Geometry: final body of the model. Coordinates: model frame, mm. A direction names the side the tool comes from. Round coordinates to 2 decimals unless told otherwise and drop trailing zeros. Order: outer loops, then holes, each group sorted by start corner. A loop starts at its lowest first (then second) coordinate and runs counter-clockwise, first axis right, second up. Notation, with made-up numbers: (88, -5.5) - (103, -5.5) arc R13 cw to (103, 7.5) - close; hole circle Ø6 at (43, -9). An arc over 180 degrees is marked (long way). Put each result on its own line as item: value. Start each with the question number.
(1) Section D-D (x = -24.2). Output: boundary loops of the cut face in (y, z) (3 decimals).
(2) Pin query (flat end, axial travel): P1, Ø3, axis at x = 24.2, z = 19.7, coming from the -Y side. Return the tip coordinate at first contact, or that it passes through.
(3) Section A-A (x = -11.5). Output: boundary loops of the cut face in (y, z), and give its area (3 significant figures).
(4) Access query for faces 4 (the face through (-17.375, 1, 0)), 5 (the face through (0, 2, -19)). Directions: +Z, -Z, +X, -X, +Y, -Y. A direction counts if a zero-diameter tool reaches every point of the face in a straight line with its end or side. Return the directions, or none.
(5) Pull-direction query (Z, two-part tool) for faces 1 (the face through (22.59, 0.99, -20.93)), 2 (the face through (29.58, 0.99, 24.89)), 3 (the face through (-33, 1, 0)); classes: released by +Z, released by -Z, zero draft, split by the parting line, or undercut.
(6) Material intervals for L1, parallel to Z at x = 23, y = 1.5; L2, parallel to X at y = 1.2, z = -8.5 (3 decimals); L3, parallel to X at y = 0.6, z = 20, sorted ascending. Write a range as [from, to].
(7) Section B-B (y = 0.9). Output: boundary loops of the cut face in (x, z) (3 decimals), and give its area (3 significant figures).
(8) Section C-C (z = 12). Output: boundary loops of the cut face in (x, y) (3 decimals), and give its area (3 significant figures).
from build123d import *

# Parameters (mm, degrees)
F0_R     = 2.025
F0_W     = 34.75
F0_H     = 31.1
F1_DEPTH = 2


with BuildPart() as f1:
    # F0 (on Front) → F1 (new body)
    with BuildSketch(Plane.XZ):
        with BuildLine():
            Line((-21, -28.5), (21, -28.5))
            ThreePointArc((21, -28.5), (29.485281, -24.985281), (33, -16.5))
            Line((33, -16.5), (33, 16.5))
            ThreePointArc((33, 16.5), (29.485281, 24.985281), (21, 28.5))
            Line((21, 28.5), (-21, 28.5))
            ThreePointArc((-21, 28.5), (-29.485281, 24.985281), (-33, 16.5))
            Line((-33, 16.5), (-33, -16.5))
            ThreePointArc((-33, -16.5), (-29.485281, -24.985281), (-21, -28.5))
        make_face()
        with Locations((-24.2, -19.7)):
            Circle(F0_R, mode=Mode.SUBTRACT)
        with Locations((24.2, -19.7)):
            Circle(F0_R, mode=Mode.SUBTRACT)
        with Locations((-24.2, 19.7)):
            Circle(F0_R, mode=Mode.SUBTRACT)
        Rectangle(F0_W, F0_H, mode=Mode.SUBTRACT)
        with Locations((24.2, 19.7)):
            Circle(F0_R, mode=Mode.SUBTRACT)
    extrude(amount=-F1_DEPTH)


solid = f1.part
Checks:
1. outline: (0, -28.065) - (2, -28.065) - (2, -21.725) - (0, -21.725) - close; (0, -17.675) - (2, -17.675) - (2, 17.675) - (0, 17.675) - close; (0, 21.725) - (2, 21.725) - (2, 28.065) - (0, 28.065) - close
2. P1: passes through
3. outline: (0, -28.5) - (2, -28.5) - (2, -15.55) - (0, -15.55) - close; (0, 15.55) - (2, 15.55) - (2, 28.5) - (0, 28.5) - close
3. area: 51.8 mm²
4. face 4: +Y, -Y
4. face 5: +Z, -Z, +X, -X, +Y
5. face 1: undercut
5. face 2: released by +Z
5. face 3: zero draft
6. L1: z = [-28.33, -21.33], [-18.07, 18.07], [21.33, 28.33]
6. L2: x = [-33, -17.375], [17.375, 33]
6. L3: x = [-32.48, -26.2], [-22.2, 22.2], [26.2, 32.48]
7. outline: (-33, -16.5) arc R12 ccw to (-21, -28.5) - (21, -28.5) arc R12 ccw to (33, -16.5) - (33, 16.5) arc R12 ccw to (21, 28.5) - (-21, 28.5) arc R12 ccw to (-33, 16.5) - close; hole circle Ø4.05 at (-24.2, -19.7); hole circle Ø4.05 at (-24.2, 19.7); hole (-17.375, -15.55) - (17.375, -15.55) - (17.375, 15.55) - (-17.375, 15.55) - close; hole circle Ø4.05 at (24.2, -19.7); hole circle Ø4.05 at (24.2, 19.7)
7. area: 2,510 mm²
8. outline: (-33, 0) - (-17.375, 0) - (-17.375, 2) - (-33, 2) - close; (17.375, 0) - (33, 0) - (33, 2) - (17.375, 2) - close
8. area: 62.5 mm²
